Can you work these out from the model? Positions are in its coordinate system, mm. Face numbers are marked on the shaded views. Give positions to 0.01 mm unless a question says otherwise; leave off trailing zeros. Loops run counter-clockwise (first coordinate to the right, second up) from the corner with the lowest first, then second, coordinate; pieces in that order, holes last. Notation, with made-up numbers: M 40.5,75.5 L 73.5,75.5 A20 cw 73.5,92.5 Z; hole C 43,42 d4. An arc over 180 degrees is marked long. Answer as a JSON object with one key per item and string values.
Autodesk Inventor part; units mm, degrees
ref_plane "YZ Plane" through (0, 0, 0) normal (1, 0, 0) x (0, 1, 0)
ref_plane "XZ Plane" through (0, 0, 0) normal (0, 1, 0) x (-1, 0, 0)
ref_plane "XY Plane" through (0, 0, 0) normal (0, 0, 1) x (1, 0, 0)
sketch "Sketch1" plane through (0, 0, 0) normal (0, 0, 1) x (1, 0, 0)
  arc A0 (19.05, 0) -> (0, 19.05) centre (0, 0) ccw
  line L0 (0, 19.05) -> (0, 0)
  line L1 (0, 0) -> (19.05, 0)
  dimension "d0" = 38.1
extrude "Extrusion1" add sketch "Sketch1" along normal mid plane 161.925
sketch "Sketch2" plane through (0, 0, 80.9625) normal (0, -1, 0) x (1, 0, 0)
  line L0 (0, -38.1) -> (4.7625, -38.1)
  line L1 (4.7625, -38.1) -> (4.7625, -123.825)
  line L2 (4.7625, -123.825) -> (0, -123.825)
  line L3 (0, -123.825) -> (0, -38.1)
  line L4 (19.05, -161.925) -> (0, -161.925)
  line L5 (0, -161.925) -> (0, 0)
  point P0 (0, -80.9625)
  dimension "d3" = 85.725
  dimension "d4" = 38.1
  dimension "d5" = 4.7625
extrude "Extrusion2" cut sketch "Sketch2" against normal through all
equation "\"d0\" = cornerRoundType"
equation "\"d1\" = lengthOfPart"
equation "\"d3\" = notchCutout"
equation "\"d4\" = bottomLength"
equation "\"d5\" = notchDepth"
equation "\"cornerRoundType\" = 38.1"
equation "\"notchCutout\" = 85.725"
equation "\"bottomLength\" = 38.1"
equation "\"lengthOfPart\" = 2 * bottomLength + notchCutout"
equation "\"notchDepth\" = 4.7625"
properties part number "topOfStairs_01875_notch"
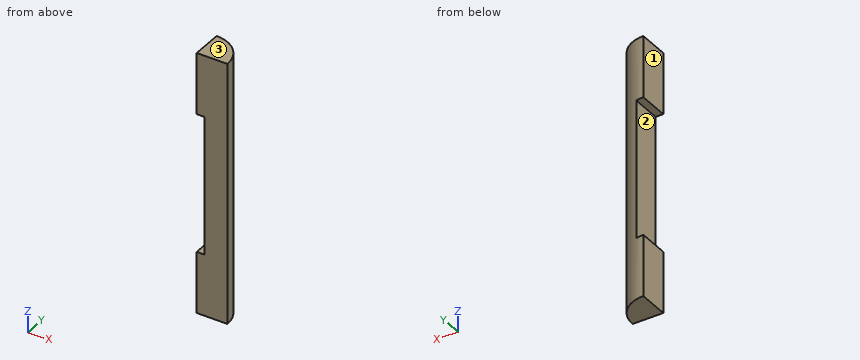
1) Suppose I cut it at C-C, the plane z = 69.5. Write out the boundary of the cut face in (x, y), and give its area (3 significant figures).
Answer list:
{"outline": "M 0,0 L 19.05,0 A19.05 ccw 0,19.05 Z", "area": "285 mm^2"}
2) Please list where these lines run through material, in increasing order: line 1 along Z through (x, y) = (1.5, 8.5); line 2 along Y through (x, z) = (1, 51); line 3 along X through (y, z) = (1, 37). Write a range as from..to.
Answer list:
{"line 1": "-80.96..-42.86, 42.86..80.96", "line 2": "0..19.02", "line 3": "4.76..19.02"}
3) Suppose I cut it at D-D, the plane y = 7.5. Write out the boundary of the cut face in (x, z), and give its area (3 significant figures).
Answer list:
{"outline": "M 0,-80.96 L 17.51,-80.96 L 17.51,80.96 L 0,80.96 L 0,42.86 L 4.76,42.86 L 4.76,-42.86 L 0,-42.86 Z", "area": "2,430 mm^2"}
4) If we mould it in two halves opening along Z, with no side actions, what happens to the marked faces 1, 2 and 3? For each: +Z half, -Z half, draft (parallel to the pull), parting line (faces both ways), or undercut.
Answer list:
{"face 1": "draft", "face 2": "undercut", "face 3": "+Z half"}
5) Suppose I cut it at B-B, the plane y = 16.25. Write out the boundary of the cut face in (x, z).
Answer list:
{"outline": "M 0,-80.96 L 9.94,-80.96 L 9.94,80.96 L 0,80.96 L 0,42.86 L 4.76,42.86 L 4.76,-42.86 L 0,-42.86 Z"}
6) Suppose I cut it at A-A, the plane x = 1.5. Write out the boundary of the cut face in (y, z), and give its area (3 significant figures).
Answer list:
{"outline": "M 0,-80.96 L 18.99,-80.96 L 18.99,-42.86 L 0,-42.86 Z; M 0,42.86 L 18.99,42.86 L 18.99,80.96 L 0,80.96 Z", "area": "1,450 mm^2"}
7) Will these pins go through, and if not, where does the flat tip stop? pin 1 Ø5 at (y, z) = (2, -18) entering from -X; pin 2 Ø8 at (y, z) = (14, 43) entering from +X; pin 3 Ø5 at (x, z) = (9, 61) entering from -Y; pin 4 Ø1 at (y, z) = (3, -38) entering from +X.
Answer list:
{"pin 1": "x = 4.76", "pin 2": "x = 16.21", "pin 3": "y = 0", "pin 4": "x = 18.89"}
